Design review of the part built by this model. Coordinates are the model's own, in mm. Face numbers are marked on the shaded views. A direction names the side the tool comes from. Coordinates: 2 decimals unless noted, no trailing zeros. Write each loop counter-clockwise with the first axis right and the second up, starting at its lowest first coordinate (ties: lowest second). Pieces come first, ordered by that corner, then holes.
Q1. For pin 1 Ø1 at (x, y) = (6.5, 0.5) entering from +Z; pin 2 Ø1.3 at (x, z) = (-2.5, -26) entering from +Y; pin 3 Ø0.8 at (x, z) = (-3.5, -25.5) entering from -Y; pin 4 Ø4 at (x, z) = (-0.5, 27.5) entering from +Y, all flat-tipped, find the tip position at first contact; note any pin that passes through.
Q2. For L1, parallel to Z at x = -4, y = -1; L2, parallel to Z at x = -6, y = -1.75; L3, parallel to Z at x = -10, y = -4.5, list the stretches that pass through material, from the lowest coordinate up.
Q3. Take a section at D-D, the plane y = 0.7. Write out the cut boundary in (x, z), plus the area to 3 significant figures.
Q4. Take a section at A-A, the plane x = 0. Write out the cut boundary in (y, z).
Q5. For the marked faces 1, 2 and 3, list the 3-axis set-ups (+Z, -Z, +X, -X, +Y, -Y) from which the entire face can be reached by the end or side of a thin tool; tool diameter is ignored.
Q6. Take a section at B-B, the plane x = -4.45. Write out the cut boundary in (y, z).
Q7. The part is to be moulded in two halves that separate along Z. For the marked faces 4 and 5, say which applies: released by +Z, released by -Z, zero draft, split by the parting line, or undercut.
Q8. Take a section at C-C, the plane z = -12.5. Write out the cut boundary in (x, y).
from build123d import *

# Parameters (mm, degrees)
ESQUISSE1_W        = 25.4
ESQUISSE1_H        = 12.5
BOSS_EXTRU_1_DEPTH = 25.25
CONG_1_R           = 4
ESQUISSE2_W        = 6.9
ESQUISSE2_H        = 1.9
BOSS_EXTRU_2_DEPTH = 1.5
ESQUISSE3_W        = 10.8
ESQUISSE3_H        = 7.2
BOSS_EXTRU_3_DEPTH = 18.6
ESQUISSE4_R        = 3.5
BOSS_EXTRU_4_DEPTH = 10.4
ESQUISSE5_R        = 2.25
BOSS_EXTRU_5_DEPTH = 10
ESQUISSE7_W        = 15
ESQUISSE7_H        = 5.6
BOSS_EXTRU_7_DEPTH = 1.6
ESQUISSE6_R        = 2.75
BOSS_EXTRU_6_DEPTH = 10


with BuildPart() as part:
    # Esquisse1 → Boss.-Extru.1 (new, symmetric)
    with BuildSketch(Plane.XY):
        Rectangle(ESQUISSE1_W, ESQUISSE1_H)
    extrude(amount=BOSS_EXTRU_1_DEPTH, both=True)

    # Congé1
    cong_1_edges = [part.edges().sort_by_distance(p)[0] for p in [
        (-12.7, 6.25, 0),
        (12.7, 6.25, 0),
        (12.7, -6.25, 0),
        (-12.7, -6.25, 0),
    ]]
    fillet(cong_1_edges, radius=CONG_1_R)

    # Esquisse2 → Boss.-Extru.2 (add)
    with BuildSketch(Plane.XY.offset(25.25)):
        with Locations((-4.45, 0.7)):
            Rectangle(ESQUISSE2_W, ESQUISSE2_H)
    extrude(amount=BOSS_EXTRU_2_DEPTH)

    # Esquisse3 → Boss.-Extru.3 (add)
    with BuildSketch(Plane.XY.offset(26.75)):
        with Locations((-4.45, 0.7)):
            Rectangle(ESQUISSE3_W, ESQUISSE3_H)
    extrude(amount=BOSS_EXTRU_3_DEPTH)

    # Esquisse4 → Boss.-Extru.4 (add)
    with BuildSketch(Plane.XY.offset(45.35)):
        with Locations((-4.45, 0.7)):
            Circle(ESQUISSE4_R)
    extrude(amount=BOSS_EXTRU_4_DEPTH)

    # Esquisse5 → Boss.-Extru.5 (add)
    with BuildSketch(Plane.XY.offset(55.75)):
        with Locations((-4.45, 0.7)):
            Circle(ESQUISSE5_R)
    extrude(amount=BOSS_EXTRU_5_DEPTH)

    # Esquisse7 → Boss.-Extru.7 (add)
    with BuildSketch(Plane(origin=(0, 0, -25.25), x_dir=(-1, 0, 0), z_dir=(0, 0, -1))):
        with Locations((0, 0.95)):
            Rectangle(ESQUISSE7_W, ESQUISSE7_H)
    extrude(amount=BOSS_EXTRU_7_DEPTH)

    # Esquisse6 → Boss.-Extru.6 (add)
    with BuildSketch(Plane(origin=(0, 0, -26.85), x_dir=(-1, 0, 0), z_dir=(0, 0, -1))):
        with Locations(Location((0, 1.25, 0), (0, 0, 114.619977329))):
            Circle(ESQUISSE6_R)
    extrude(amount=BOSS_EXTRU_6_DEPTH)


solid = part.part
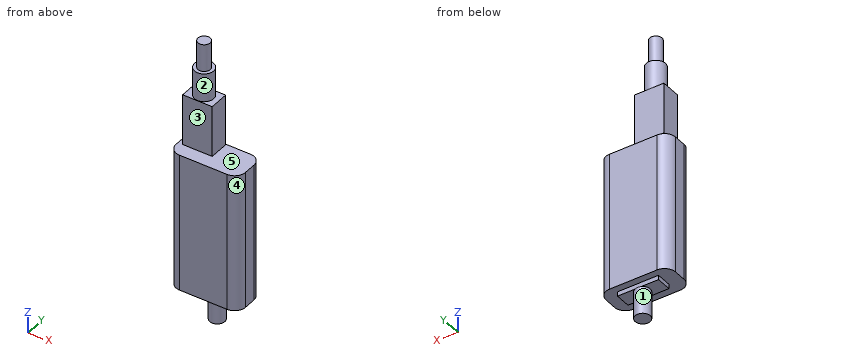
Responses:
1. pin 1: stops at z = 25.25
1. pin 2: stops at y = 3.75
1. pin 3: stops at y = -6.25
1. pin 4: stops at y = 4.3
2. L1: z = -26.85 to 25.25, 26.75 to 65.75
2. L2: z = -26.85 to 25.25, 26.75 to 55.75
2. L3: z = -25.25 to 25.25
3. outline: (-12.7, -25.25) - (-7.5, -25.25) - (-7.5, -26.85) - (-2.69, -26.85) - (-2.69, -36.85) - (2.69, -36.85) - (2.69, -26.85) - (7.5, -26.85) - (7.5, -25.25) - (12.7, -25.25) - (12.7, 25.25) - (-1, 25.25) - (-1, 26.75) - (0.95, 26.75) - (0.95, 45.35) - (-0.95, 45.35) - (-0.95, 55.75) - (-2.2, 55.75) - (-2.2, 65.75) - (-6.7, 65.75) - (-6.7, 55.75) - (-7.95, 55.75) - (-7.95, 45.35) - (-9.85, 45.35) - (-9.85, 26.75) - (-7.9, 26.75) - (-7.9, 25.25) - (-12.7, 25.25) - close
3. area: 1,690 mm2
4. outline: (-6.25, -25.25) - (-1.85, -25.25) - (-1.85, -26.85) - (-1.5, -26.85) - (-1.5, -36.85) - (4, -36.85) - (4, -26.85) - (3.75, -26.85) - (3.75, -25.25) - (6.25, -25.25) - (6.25, 25.25) - (-6.25, 25.25) - close; (-2.9, 26.75) - (4.3, 26.75) - (4.3, 45.35) - (-2.9, 45.35) - close
5. face 1: -Z
5. face 2: +Z
5. face 3: +Z, +X, -X, -Y
6. outline: (-6.25, -25.25) - (-1.85, -25.25) - (-1.85, -26.85) - (3.75, -26.85) - (3.75, -25.25) - (6.25, -25.25) - (6.25, 25.25) - (1.65, 25.25) - (1.65, 26.75) - (4.3, 26.75) - (4.3, 45.35) - (4.2, 45.35) - (4.2, 55.75) - (2.95, 55.75) - (2.95, 65.75) - (-1.55, 65.75) - (-1.55, 55.75) - (-2.8, 55.75) - (-2.8, 45.35) - (-2.9, 45.35) - (-2.9, 26.75) - (-0.25, 26.75) - (-0.25, 25.25) - (-6.25, 25.25) - close
7. face 4: zero draft
7. face 5: undercut
8. outline: (-12.7, -2.25) arc R4 ccw to (-8.7, -6.25) - (8.7, -6.25) arc R4 ccw to (12.7, -2.25) - (12.7, 2.25) arc R4 ccw to (8.7, 6.25) - (-8.7, 6.25) arc R4 ccw to (-12.7, 2.25) - close
